from build123d import *

# Parameters (mm, degrees)
SKETCH1_R           = 1.7
SKETCH1_W           = 10
SKETCH1_H           = 12.5
BOSS_EXTRUDE1_DEPTH = 2.5
SKETCH2_W           = 5
SKETCH2_H           = 16
BOSS_EXTRUDE2_DEPTH = 2.5
SKETCH3_W           = 1.7
SKETCH3_H           = 5
CUT_EXTRUDE1_DEPTH  = 29.940283343
SKETCH6_R           = 1.59
CUT_EXTRUDE3_DEPTH  = 16.7
BOSS_EXTRUDE3_DEPTH = 3.5
BOSS_EXTRUDE5_DEPTH = 3.5
SKETCH10_R          = 4
BOSS_EXTRUDE6_DEPTH = 1.875
SKETCH11_R          = 1.7
CUT_EXTRUDE4_DEPTH  = 30.481567746
SKETCH12_R          = 4
CUT_EXTRUDE5_DEPTH  = 1
FILLET1_R           = 1
FILLET2_R           = 1
FILLET3_R           = 0.25
FILLET4_R           = 0.25


with BuildPart() as part:
    # Sketch1 → Boss-Extrude1 (new body)
    # profile 1 of 2: a face of its own
    with BuildSketch(Plane.XY):
        with BuildLine():
            ThreePointArc((0, 6.25), (-6.25, 0), (0, -6.25))
            Line((0, -6.25), (12.7, -6.25))
            Line((12.7, -6.25), (12.7, 6.25))
            Line((12.7, 6.25), (0, 6.25))
        make_face()
        Circle(SKETCH1_R, mode=Mode.SUBTRACT)
    # profile 2 of 2: a face of its own
    with BuildSketch(Plane.XY):
        with Locations((17.7, 0)):
            Rectangle(SKETCH1_W, SKETCH1_H)
    extrude(amount=BOSS_EXTRUDE1_DEPTH)

    # Sketch2 → Boss-Extrude2 (add)
    with BuildSketch(Plane.XY.offset(2.5)):
        with Locations((25.2, 0)):
            Rectangle(SKETCH2_W, SKETCH2_H)
    extrude(amount=-BOSS_EXTRUDE2_DEPTH)

    # Sketch3 → Cut-Extrude1 (cut, through all)
    with BuildSketch(Plane.XY.offset(2.5)):
        with Locations((21.85, 0)):
            Rectangle(SKETCH3_W, SKETCH3_H)
    extrude(amount=-CUT_EXTRUDE1_DEPTH, mode=Mode.SUBTRACT)

    # Sketch6 → Cut-Extrude3 (cut)
    with BuildSketch(Plane(origin=(27.7, 0, 0), x_dir=(0, 0, -1), z_dir=(1, 0, 0))):
        with Locations((-1.25, 0)):
            Circle(SKETCH6_R)
    extrude(amount=-CUT_EXTRUDE3_DEPTH, mode=Mode.SUBTRACT)


with BuildPart() as body_2:
    # Sketch7 → Boss-Extrude3 (new body)
    with BuildSketch(Plane.XZ.offset(6.25)):
        with BuildLine():
            Line((6.129900512, 3.210673711), (6.129900512, 4.710673711))
            ThreePointArc((6.129900512, 4.710673711), (6.694341527, 4.327552018), (7.360579964, 4.180915603))
            ThreePointArc((7.360579964, 4.180915603), (7.789326283, 4.199870579), (8.206709695, 4.299739418))
            ThreePointArc((8.206709695, 4.299739418), (15.494742209, 6.151071465), (22.7, 4))
            Line((22.7, 4), (22.7, 2.5))
            ThreePointArc((22.7, 2.5), (15.494742209, 4.651071465), (8.206709695, 2.799739418))
            ThreePointArc((8.206709695, 2.799739418), (7.789326283, 2.699870579), (7.360579964, 2.680915603))
            ThreePointArc((7.360579964, 2.680915603), (6.694341527, 2.827552018), (6.129900512, 3.210673711))
        make_face()
    extrude(amount=-BOSS_EXTRUDE3_DEPTH)


with BuildPart() as body_3:
    # Sketch9 → Boss-Extrude5 (new body)
    with BuildSketch(Plane.XZ.offset(6.25)):
        Polygon((22.7, 4), (25.104907101, 2.5), (22.7, 2.5), align=None)
    extrude(amount=-BOSS_EXTRUDE5_DEPTH)

    # Combine1: union body 2
    add(body_2.part)


with BuildPart() as body_3_2:
    # Mirror5: mirrored copy
    add(body_3.part.mirror(Plane(origin=(0, 0, 0), x_dir=(0, 0, 1), z_dir=(0, -1, 0))))


with BuildPart() as part_1:
    add(part.part)

    # Combine4: union body 3, body 3 2
    add(body_3.part)
    add(body_3_2.part)

    # Sketch10 → Boss-Extrude6 (add)
    with BuildSketch(Plane(origin=(0, 0, 0), x_dir=(-1, 0, 0), z_dir=(0, 0, -1))):
        with Locations(Location((0, 0, 0), (0, 0, 180))):
            Circle(SKETCH10_R)
    extrude(amount=BOSS_EXTRUDE6_DEPTH)

    # Sketch11 → Cut-Extrude4 (cut, through all)
    with BuildSketch(Plane.XY):
        Circle(SKETCH11_R)
    extrude(amount=-CUT_EXTRUDE4_DEPTH, mode=Mode.SUBTRACT)

    # Sketch12 → Cut-Extrude5 (cut)
    with BuildSketch(Plane.XY.offset(2.5)):
        Circle(SKETCH12_R)
    extrude(amount=-CUT_EXTRUDE5_DEPTH, mode=Mode.SUBTRACT)

    # Fillet1
    fillet1_edges = [part_1.edges().sort_by_distance(p)[0] for p in [
        (-4, 0, 2.5),
    ]]
    fillet(fillet1_edges, radius=FILLET1_R - 0.0001)  # a hair under: the kernel refuses the full size

    # Fillet2
    fillet2_edges = [part_1.edges().sort_by_distance(p)[0] for p in [
        (-4, 0, -1.875),
    ]]
    fillet(fillet2_edges, radius=FILLET2_R)

    # Fillet3
    fillet3_edges = [part_1.edges().sort_by_distance(p)[0] for p in [
        (16, 0.98264948, 2.5),
        (16, -0.98264948, 2.5),
        (16, 0.98264948, 0),
        (16, -0.98264948, 0),
    ]]
    fillet(fillet3_edges, radius=FILLET3_R)

    # Fillet4
    fillet4_edges = [part_1.edges().sort_by_distance(p)[0] for p in [
        (25.2, 0.98264948, 2.5),
        (25.2, -0.98264948, 2.5),
        (25.2, 0.98264948, 0),
        (25.2, -0.98264948, 0),
    ]]
    fillet(fillet4_edges, radius=FILLET4_R)


solid = part_1.part
CAD build for the part. Positions are in the model's coordinates, mm. A direction names the side the tool comes from. Round coordinates to 2 decimals unless told otherwise and drop trailing zeros. Order: outer loops, then holes, each group sorted by start corner. A loop starts at its lowest first (then second) coordinate and runs counter-clockwise, first axis right, second up. Notation, with made-up numbers: (0.25, 45) -> (39.25, 45) arc R33 cw to (39.25, 78) -> close; hole circle Ø4 at (63.5, -23.75). An arc over 180 degrees is marked (long way). Write each question's results on one line, items separated by ' | '.
1. Cut at B-B (x = 19). Give the cut face in (y, z).
Findings below:
outline: (-6.25, 0) -> (-1.54, 0) arc R0.25 ccw to (-1.33, 0.39) arc R1.59 cw to (-1.33, 2.11) arc R0.25 ccw to (-1.54, 2.5) -> (-6.25, 2.5) -> close; (-6.25, 4.13) -> (-2.75, 4.13) -> (-2.75, 5.63) -> (-6.25, 5.63) -> close; (1.33, 0.39) arc R0.25 ccw to (1.54, 0) -> (6.25, 0) -> (6.25, 2.5) -> (1.54, 2.5) arc R0.25 ccw to (1.33, 2.11) arc R1.59 cw to start; (2.75, 4.13) -> (6.25, 4.13) -> (6.25, 5.63) -> (2.75, 5.63) -> close
2. Wall check: line 1 along Y through (x, z) = (8.5, 3); line 2 along Y through (x, z) = (0, -0.85); line 3 along Z through (x, y) = (15.5, -6). Give the ranges that are in metal, low to high. Write a range as [from, to].
Findings below:
line 1: y = [-6.25, -2.75], [2.75, 6.25] | line 2: y = [-4, -1.7], [1.7, 4] | line 3: z = [0, 2.5], [4.65, 6.15]
3. Cut at C-C (x = 9.5). Give the cut face in (y, z).
Findings below:
outline: (-6.25, 0) -> (6.25, 0) -> (6.25, 2.5) -> (-6.25, 2.5) -> close; (-6.25, 3.45) -> (-2.75, 3.45) -> (-2.75, 4.95) -> (-6.25, 4.95) -> close; (2.75, 3.45) -> (6.25, 3.45) -> (6.25, 4.95) -> (2.75, 4.95) -> close
4. Pull direction Y, two halves, no side cores. Call faces 4 (the face through (21, -2, 1)), 5 (the face through (25, 8, 1)), 6 (the face through (6.69, 4.52, 4.33)): pulls with the +Y half, pulls with the -Y half, needs draft (parallel to the pull), parting line crosses it, or undercut.
Findings below:
face 4: undercut | face 5: pulls with the +Y half | face 6: needs draft
5. 3-axis set-ups, long thin cutter, end or side, ignore diameter. For faces 1 (the face through (25.24, 1.59, 1.24)), 2 (the face through (22.7, 2, 1)), 3 (the face through (6.13, -5, 4)): which of +Z, -Z, +X, -X, +Y, -Y reach the whole face in a straight line?
Findings below:
face 1: +X | face 2: +Z, -Z | face 3: +Z, -X, +Y, -Y
6. Flat gauge pins, fed straight in: P1, Ø3, axis at x = 15, z = 2, coming from the +Y side; P2, Ø1, axis at x = 18, y = -4.5, coming from the -Z side; P3, Ø1.2, axis at y = 4.5, z = 4, coming from the -X side. Where does each tip first touch, or does it go through?
Findings below:
P1: stops at y = 6.25 | P2: stops at z = 0 | P3: stops at x = 6.13
